Verification items for the finished model (mm, model axes). A direction names the side the tool comes from. Give positions to 0.01 mm unless a question says otherwise; leave off trailing zeros. Write each loop counter-clockwise with the first axis right and the second up, starting at its lowest first coordinate (ties: lowest second). Pieces come first, ordered by that corner, then holes. Notation, with made-up numbers: (69, -26.75) - (102, -26.75) arc R32 cw to (102, 10.25) - close; hole circle Ø3 at (39, 78). An arc over 180 degrees is marked (long way). Answer as a JSON object with one key per item and string values. Group by question number.
Item 1: Sectioned sample at D-D, the plane x = -25. Record the boundary of the cut face in (y, z) (3 decimals), and give its area (3 significant figures).
Item 2: Sectioned sample at A-A, the plane x = 0. Record the boundary of the cut face in (y, z) (3 decimals), and give its area (3 significant figures).
Item 3: Sectioned sample at C-C, the plane z = 21. Record the boundary of the cut face in (x, y), and give its area (3 significant figures).
Item 4: Sectioned sample at B-B, the plane y = 0. Record the boundary of the cut face in (x, z) (3 decimals), and give its area (3 significant figures).
Item 5: Draft check along X on faces 1 (the face through (-2.75, -12.4, 18.96)), 2 (the face through (44.45, 0, -3)), 3 (the face through (0, 28.575, 6)). Enter one of: +X half, -X half, draft (parallel to the pull), parting line (faces both ways), or undercut.
Item 6: Tool access check on faces 4 (the face through (-28.575, 0, 6)), 5 (the face through (28.575, 0, 6)), 6 (the face through (0, -28.575, 6)), 7 (the face through (0, 0, 12.7)). Record the directions out of +Z, -Z, +X, -X, +Y, -Y that give a thin tool (end or side, any length) a straight path to the whole face; none if there is none.
Item 7: Scan lines: line 1 along Y through (x, z) = (0, 17.25); line 2 along Z through (x, y) = (36.5, 1); line 3 along X through (y, z) = (-8.5, 10) (3 decimals). Record each from-to range of solid material in increasing order. Write a range as [from, to].
Item 8: Go/stop test with flat-tipped pins: pin 1 (6.5 mm diameter, centred on y = -4, z = 4.5, fed in from +X) (3 decimals); pin 2 (8 mm diameter, centred on x = 19.5, z = 5.5, fed in from -Y) (3 decimals); pin 3 (6.5 mm diameter, centred on y = -8.5, z = 9.5, fed in from -X) (3 decimals); pin 4 (1.5 mm diameter, centred on x = -29, z = 14, fed in from +Y). Record where each tip stops, or that it passes through.
```python
from build123d import *

# Parameters (mm, degrees)
SKETCH2_W           = 88.9
SKETCH2_H           = 63.5
BOSS_EXTRUDE1_DEPTH = 6.35
SKETCH3_W           = 57.15
SKETCH3_H           = 57.15
BOSS_EXTRUDE2_DEPTH = 12.7
SKETCH4_R           = 19.05
SKETCH4_R_2         = 12.7
BOSS_EXTRUDE3_DEPTH = 12.7


with BuildPart() as part:
    # Sketch2 → Boss-Extrude1 (new body)
    with BuildSketch(Plane.XY):
        Rectangle(SKETCH2_W, SKETCH2_H)
    extrude(amount=-BOSS_EXTRUDE1_DEPTH)

    # Sketch3 → Boss-Extrude2 (add)
    with BuildSketch(Plane.XY):
        Rectangle(SKETCH3_W, SKETCH3_H)
    extrude(amount=BOSS_EXTRUDE2_DEPTH)

    # Sketch4 → Boss-Extrude3 (add)
    with BuildSketch(Plane.XY.offset(12.7)):
        Circle(SKETCH4_R)
        Circle(SKETCH4_R_2, mode=Mode.SUBTRACT)
    extrude(amount=BOSS_EXTRUDE3_DEPTH)


solid = part.part
```
Geometry check:
{
 "1": {"outline": "(-31.75, -6.35) - (31.75, -6.35) - (31.75, 0) - (28.575, 0) - (28.575, 12.7) - (-28.575, 12.7) - (-28.575, 0) - (-31.75, 0) - close", "area": "1,130 mm^2"},
 "2": {"outline": "(-31.75, -6.35) - (31.75, -6.35) - (31.75, 0) - (28.575, 0) - (28.575, 12.7) - (19.05, 12.7) - (19.05, 25.4) - (12.7, 25.4) - (12.7, 12.7) - (-12.7, 12.7) - (-12.7, 25.4) - (-19.05, 25.4) - (-19.05, 12.7) - (-28.575, 12.7) - (-28.575, 0) - (-31.75, 0) - close", "area": "1,290 mm^2"},
 "3": {"outline": "circle Ø38.1 at (0, 0); hole circle Ø25.4 at (0, 0)", "area": "633 mm^2"},
 "4": {"outline": "(-44.45, -6.35) - (44.45, -6.35) - (44.45, 0) - (28.575, 0) - (28.575, 12.7) - (19.05, 12.7) - (19.05, 25.4) - (12.7, 25.4) - (12.7, 12.7) - (-12.7, 12.7) - (-12.7, 25.4) - (-19.05, 25.4) - (-19.05, 12.7) - (-28.575, 12.7) - (-28.575, 0) - (-44.45, 0) - close", "area": "1,450 mm^2"},
 "5": {"face 1": "undercut", "face 2": "+X half", "face 3": "draft"},
 "6": {"face 4": "+Z, -X, +Y, -Y", "face 5": "+Z, +X, +Y, -Y", "face 6": "+Z, +X, -X, -Y", "face 7": "+Z"},
 "7": {"line 1": "[-19.05, -12.7], [12.7, 19.05]", "line 2": "[-6.35, 0]", "line 3": "[-28.575, 28.575]"},
 "8": {"pin 1": "x = 28.575", "pin 2": "y = -28.575", "pin 3": "x = -28.575", "pin 4": "through"}
}
